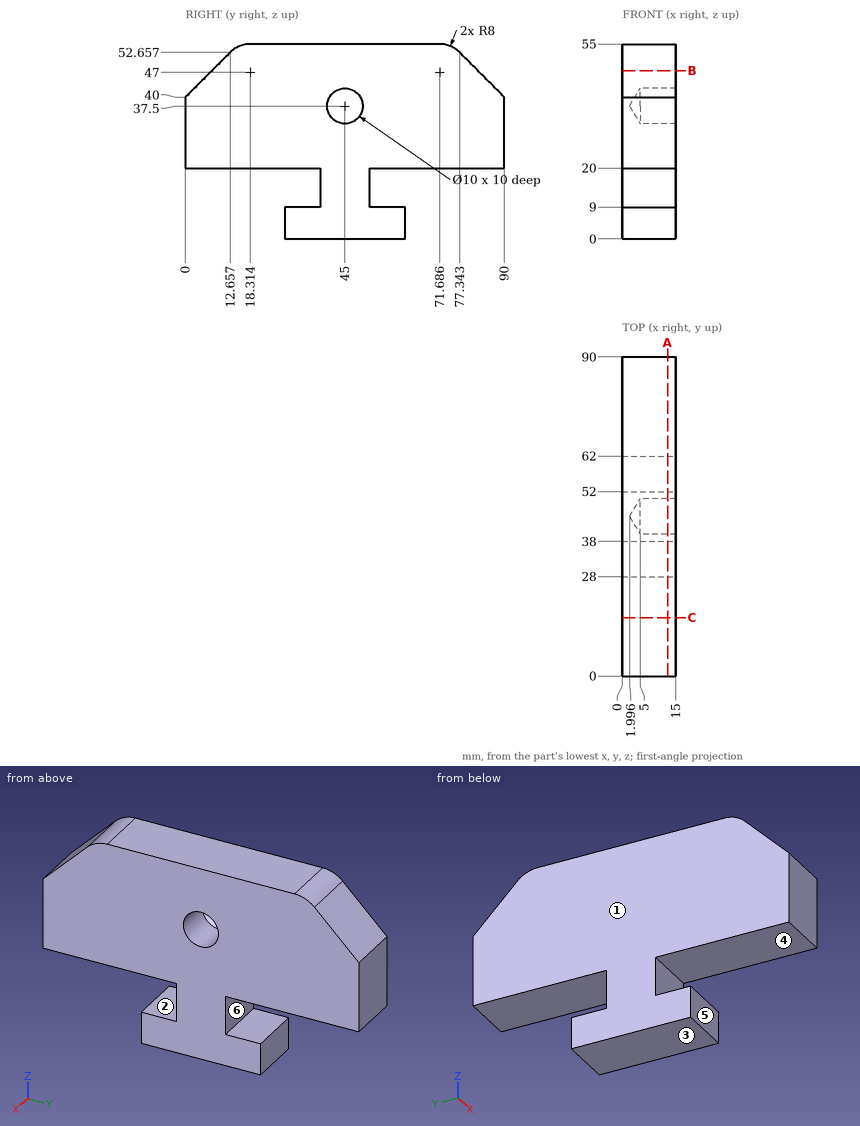
Input: dimensioned drawing with shaded views. Units: mm. Origin: part minimum x, y, z. A direction names the side the tool comes from. Round coordinates to 2 decimals unless told otherwise and drop trailing zeros. Order: outer loops, then holes, each group sorted by start corner. A loop starts at its lowest first (then second) coordinate and runs counter-clockwise, first axis right, second up. Notation, with made-up numbers: (-10.75, -19) -> (4.25, -19) arc R23 ccw to (4.25, 5) -> close; hole circle Ø9 at (-37.75, 21). An arc over 180 degrees is marked (long way). One line per item, written item: value. Start each with the question number.
Q1. Section query C-C (y = 16.5). Return the cut outline in (x, z), plus the area to 3 significant figures.
Q2. Section query A-A (x = 12.75). Return the cut outline in (y, z).
Q3. Material intervals for probe 1 along Y at (x, z) = (13, 37.5); probe 2 along Z at (x, y) = (11, 45); probe 3 along Z at (x, y) = (1.25, 28.5), sorted ascending.
Q4. Draft query along Z for the marked faces 1, 2 and 3. Return one class per face: pulls with the +Z half, pulls with the -Z half, needs draft (parallel to the pull), parting line crosses it, or undercut.
Q5. Access query for the marked faces 4, 5 and 6. Directions: +Z, -Z, +X, -X, +Y, -Y. A direction counts if a zero-diameter tool reaches every point of the face in a straight line with its end or side. Return the directions, or none.
Q6. Pin query (flat end, axial travel): pin 1 (3.5 mm diameter, centred on x = 10, z = 13.5, fed in from +Y); pin 2 (2.5 mm diameter, centred on x = 6, z = 4, fed in from +Y); pin 3 (4.5 mm diameter, centred on x = 9.5, y = 79, fed in from -Z). Return the tip coordinate at first contact, or that it passes through.
Q7. Section query B-B (z = 47.5). Return the cut outline in (x, y).
Findings below:
1. outline: (0, 20) -> (15, 20) -> (15, 54.79) -> (0, 54.79) -> close
1. area: 522 mm²
2. outline: (0, 20) -> (38, 20) -> (38, 9) -> (28, 9) -> (28, 0) -> (62, 0) -> (62, 9) -> (52, 9) -> (52, 20) -> (90, 20) -> (90, 40) -> (77.34, 52.66) arc R8 ccw to (71.69, 55) -> (18.31, 55) arc R8 ccw to (12.66, 52.66) -> (0, 40) -> close; hole circle Ø10 at (45, 37.5)
3. probe 1: 0 to 40, 50 to 90
3. probe 2: 0 to 32.5, 42.5 to 55
3. probe 3: 0 to 9, 20 to 55
4. face 1: needs draft
4. face 2: undercut
4. face 3: pulls with the -Z half
5. face 4: +X, -X, -Y
5. face 5: -Z, +X, -X, -Y
5. face 6: +X, -X, +Y
6. pin 1: y = 52
6. pin 2: y = 62
6. pin 3: z = 20
7. outline: (0, 7.5) -> (15, 7.5) -> (15, 82.5) -> (0, 82.5) -> close
